Could you check a few things on this drawing? It's one solid part, dimensions in mm from its lowest x, y, z. A direction names the side the tool comes from. Give positions to 0.01 mm unless a question says otherwise; leave off trailing zeros. Order: outer loops, then holes, each group sorted by start corner. A loop starts at its lowest first (then second) coordinate and runs counter-clockwise, first axis right, second up.
(1) If I drill on probe 1 along Z at (x, y) = (44.25, 10); probe 2 along Y at (x, z) = (41, 37.7); probe 3 along Z at (x, y) = (12, 11), over which ranges is the centre line in solid material (lowest first)?
(2) Imagine slicing it at B-B, the plane x = 41.5. Write out the boundary of the cut face in (y, z).
(3) Imagine slicing it at D-D, the plane x = 3.5. Write out the boundary of the cut face in (y, z).
(4) Will these pins go through, and if not, where does the flat tip stop? pin 1 (12 mm diameter, centred on y = 4.5, z = 50, fed in from -X); pin 2 (7 mm diameter, centred on y = 10, z = 7.7, fed in from -X) (1 decimal); pin 3 (5 mm diameter, centred on y = 9, z = 37, fed in from -X); pin 4 (3 mm diameter, centred on y = 10, z = 37.7, fed in from +X).
(5) Imagine slicing it at A-A, the plane y = 17.25. Write out the boundary of the cut face in (x, z).
(6) On a 3-axis mill with a long thin cutter (end or side, diameter ignored), from which of +Z, -Z, +X, -X, +Y, -Y can I reach the whole of each face in a straight line? I mean the marked faces 1 and 2. Say none if no direction works.
(7) Imagine slicing it at C-C, the plane z = 46.5. Write out the boundary of the cut face in (x, y), then the cut area to 3 significant figures.
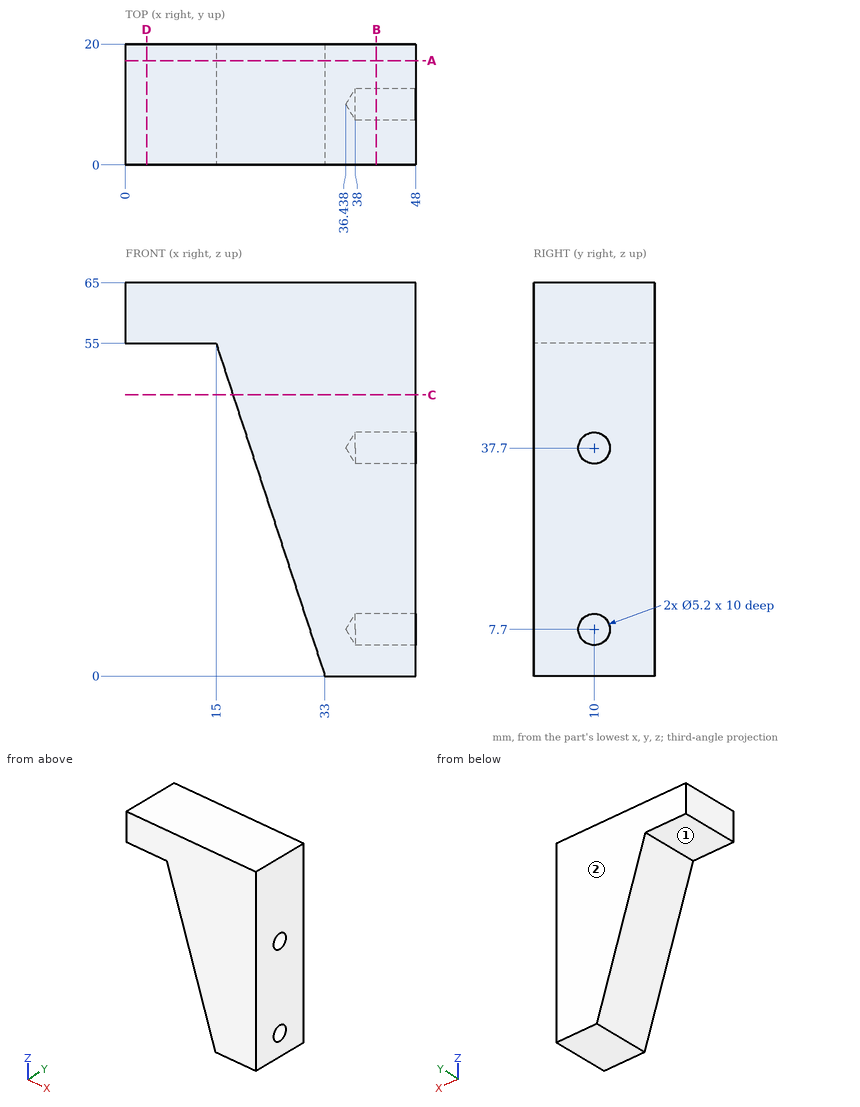
Answer block:
1. probe 1: z = 0 to 5.1, 10.3 to 35.1, 40.3 to 65
1. probe 2: y = 0 to 7.4, 12.6 to 20
1. probe 3: z = 55 to 65
2. outline: (0, 0) - (20, 0) - (20, 65) - (0, 65) - close; hole circle Ø5.2 at (10, 7.7); hole circle Ø5.2 at (10, 37.7)
3. outline: (0, 55) - (20, 55) - (20, 65) - (0, 65) - close
4. pin 1: stops at x = 0
4. pin 2: stops at x = 29.3
4. pin 3: stops at x = 20.07
4. pin 4: stops at x = 37.34
5. outline: (0, 55) - (15, 55) - (33, 0) - (48, 0) - (48, 65) - (0, 65) - close
6. face 1: -Z, -X, +Y, -Y
6. face 2: +Z, -Z, +X, -X, +Y
7. outline: (17.78, 0) - (48, 0) - (48, 20) - (17.78, 20) - close
7. area: 604 mm2
